from build123d import *

# Parameters (mm, degrees)
SKETCH1_R          = 13.062040361
SKETCH1_R_2        = 2.413
SKETCH1_W          = 134.896048872
SKETCH1_H          = 170.361865006
SKETCH1_W_2        = 8.101943593
SKETCH1_H_2        = 18.586811772
BASE_EXTRUDE_DEPTH = 3.175


with BuildPart() as part:
    # Sketch1 → Base-Extrude (new body)
    with BuildSketch(Plane.XY):
        with BuildLine():
            Line((67.448024436, -180.870824712), (80.875311853, -180.870824712))
            ThreePointArc((80.875311853, -180.870824712), (82.671363078, -180.126875936), (83.415311853, -178.330824712))
            Line((83.415311853, -178.330824712), (83.415311853, 181.634401419))
            ThreePointArc((83.415311853, 181.634401419), (82.671363078, 183.430452643), (80.875311853, 184.174401419))
            Line((80.875311853, 184.174401419), (67.448024436, 184.174401419))
            Line((67.448024436, 184.174401419), (-80.875311853, 184.174401419))
            ThreePointArc((-80.875311853, 184.174401419), (-82.671363078, 183.430452643), (-83.415311853, 181.634401419))
            Line((-83.415311853, 181.634401419), (-83.415311853, 177.378670652))
            ThreePointArc((-83.415311853, 177.378670652), (-85.086906608, 174.158747039), (-83.415311853, 170.938823426))
            Line((-83.415311853, 170.938823426), (-83.415311853, 67.926183644))
            ThreePointArc((-83.415311853, 67.926183644), (-85.086906608, 64.706260031), (-83.415311853, 61.486336418))
            Line((-83.415311853, 61.486336418), (-83.415311853, -178.330824712))
            ThreePointArc((-83.415311853, -178.330824712), (-82.671363078, -180.126875936), (-80.875311853, -180.870824712))
            Line((-80.875311853, -180.870824712), (-67.448024436, -180.870824712))
            Line((-67.448024436, -180.870824712), (-67.448024436, -172.061286826))
            Line((-67.448024436, -172.061286826), (67.448024436, -172.061286826))
            Line((67.448024436, -172.061286826), (67.448024436, -180.870824712))
        make_face()
        with Locations((-45.925033829, 18.948035519)):
            Circle(SKETCH1_R, mode=Mode.SUBTRACT)
        with Locations((-81.149906608, 174.158747039)):
            Circle(SKETCH1_R_2, mode=Mode.SUBTRACT)
        with Locations((-72.033370308, -0.104595883)):
            Circle(SKETCH1_R_2, mode=Mode.SUBTRACT)
        with Locations((-72.033370308, -160.140032971)):
            Circle(SKETCH1_R_2, mode=Mode.SUBTRACT)
        with Locations((72.033370308, -160.140032971)):
            Circle(SKETCH1_R_2, mode=Mode.SUBTRACT)
        with Locations((72.033370308, 174.158747039)):
            Circle(SKETCH1_R_2, mode=Mode.SUBTRACT)
        with Locations((72.033370308, 64.706260031)):
            Circle(SKETCH1_R_2, mode=Mode.SUBTRACT)
        with Locations((72.033370308, -0.104595883)):
            Circle(SKETCH1_R_2, mode=Mode.SUBTRACT)
        with Locations((-81.149906608, 64.706260031)):
            Circle(SKETCH1_R_2, mode=Mode.SUBTRACT)
        with BuildLine():
            Line((67.448024436, 180.158408435), (67.448024436, 38.374253759))
            Line((67.448024436, 38.374253759), (-79.118458404, 38.374253759))
            Line((-79.118458404, 38.374253759), (-79.118458404, 61.333844399))
            ThreePointArc((-79.118458404, 61.333844399), (-78.309050002, 61.980548611), (-77.696370086, 62.816007537))
            Line((-77.696370086, 62.816007537), (-77.696370086, 66.596512525))
            ThreePointArc((-77.696370086, 66.596512525), (-78.309050002, 67.431971452), (-79.118458404, 68.078675663))
            Line((-79.118458404, 68.078675663), (-79.118458404, 170.786331407))
            ThreePointArc((-79.118458404, 170.786331407), (-78.634491656, 171.130107638), (-78.207715157, 171.542742745))
            Line((-78.207715157, 171.542742745), (-78.207715157, 176.774751333))
            ThreePointArc((-78.207715157, 176.774751333), (-78.634491656, 177.18738644), (-79.118458404, 177.531162671))
            Line((-79.118458404, 177.531162671), (-79.118458404, 180.158408435))
            Line((-79.118458404, 180.158408435), (67.448024436, 180.158408435))
        make_face(mode=Mode.SUBTRACT)
        with Locations((0, -82.475585381)):
            Rectangle(SKETCH1_W, SKETCH1_H, mode=Mode.SUBTRACT)
        with Locations((-68.175247928, 23.913375939)):
            Rectangle(SKETCH1_W_2, SKETCH1_H_2, mode=Mode.SUBTRACT)
    extrude(amount=-BASE_EXTRUDE_DEPTH)


solid = part.part
The listing builds one solid part. Answer for the finished solid, in the listing's coordinates (mm). Round coordinates to 2 decimals unless told otherwise and drop trailing zeros. Write each loop counter-clockwise with the first axis right and the second up, starting at its lowest first coordinate (ties: lowest second). Pieces come first, ordered by that corner, then holes. Notation, with made-up numbers: (-33.75, -5.75) - (-25.75, -5.75) arc R6 cw to (-25.75, 0.25) - close; hole circle Ø2 at (-35.5, 76). An arc over 180 degrees is marked (long way). Use one line per item in the form item = value. Start each with the question number.
Item 1: A cutting plane is placed at D-D (z = -1.5). Give the number of separate pieces and of enclosed holes in the cut face, plus the area to 3 significant figures.
Item 2: Determine the mould class of faces 1 (the flat face through (5, 16, -3.175)), 2 (the cylindrical face through (-39.9, 7.36, -1.57)) for opening direction Y: +Y half, -Y half, draft (parallel to the pull), parting line (faces both ways), or undercut.
Item 3: A cutting plane is placed at A-A (y = -13.5). Write down the section's boundary in (x, z) (3 decimals).
Item 4: A cutting plane is placed at B-B (x = 40). Write down the section's boundary in (y, z) (3 decimals).
Item 5: Flat-ended cylindrical pins translate along their axes: pin 1 Ø1.6 at (y, z) = (-176.5, -1) entering from -X; pin 2 Ø1.5 at (x, z) = (-40.5, -0.5) entering from -Y; pin 3 Ø4 at (x, y) = (72.03, -0.1) entering from +Z. Find the tip coordinate at first contact, or state that the pin passes through.
Item 6: Find the intervals of material crossed by line 1 (Y direction, x = 52, z = -1.45); line 2 (Y direction, x = -72, z = -2.75); line 3 (X direction, y = -95, z = -2.4), in increasing order. Write a range as [from, to].
Item 7: A cutting plane is placed at C-C (x = -42). Write down the section's boundary in (y, z) (3 decimals).
The answers:
q1.separate_pieces = 1
q1.enclosed_holes = 12
q1.area = 15,100 mm^2
q2.face_1 = draft
q2.face_2 = undercut
q3.outline = (-83.415, -3.175) - (-67.448, -3.175) - (-67.448, 0) - (-83.415, 0) - close; (67.448, -3.175) - (83.415, -3.175) - (83.415, 0) - (67.448, 0) - close
q4.outline = (-172.061, -3.175) - (-167.657, -3.175) - (-167.657, 0) - (-172.061, 0) - close; (2.705, -3.175) - (38.374, -3.175) - (38.374, 0) - (2.705, 0) - close; (180.158, -3.175) - (184.174, -3.175) - (184.174, 0) - (180.158, 0) - close
q5.pin_1 = -83.42
q5.pin_2 = -172.06
q5.pin_3 = through
q6.line_1 = [-172.06, -167.66], [2.71, 38.37], [180.16, 184.17]
q6.line_2 = [-180.87, -162.55], [-157.73, -2.52], [2.31, 14.62], [33.21, 38.37], [180.16, 184.17]
q6.line_3 = [-83.42, -67.45], [67.45, 83.42]
q7.outline = (-172.061, -3.175) - (-167.657, -3.175) - (-167.657, 0) - (-172.061, 0) - close; (2.705, -3.175) - (6.49, -3.175) - (6.49, 0) - (2.705, 0) - close; (31.406, -3.175) - (38.374, -3.175) - (38.374, 0) - (31.406, 0) - close; (180.158, -3.175) - (184.174, -3.175) - (184.174, 0) - (180.158, 0) - close
